Part model, mm, in its own coordinate system. Face numbers are marked on the shaded views. A direction names the side the tool comes from. Round coordinates to 2 decimals unless told otherwise and drop trailing zeros. Write each loop counter-clockwise with the first axis right and the second up, starting at its lowest first coordinate (ties: lowest second). Pieces come first, ordered by that corner, then holes. Notation, with made-up numbers: M -1,-37.5 L 55,-37.5 A17 cw 55,-27.5 Z; hole C -37,35 d5. An arc over 180 degrees is marked long. Answer as a JSON object with one key per item and string values. Group by question number.
1. Band-saw the part on D-D, the plane z = 25.5. Write the cut outline in (x, y).
2. Drop flat-ended pins along their axis: pin 1 (2 mm diameter, centred on x = -17.5, y = -7, fed in from +Z); pin 2 (1.5 mm diameter, centred on x = -1, z = 5.5, fed in from +Y); pin 3 (1.4 mm diameter, centred on y = 6.5, z = 31, fed in from -X); pin 4 (2.5 mm diameter, centred on x = -9.525, z = 15, fed in from -Y). Give the stop position or say it passes through.
3. Drill centre lines: line 1 (X direction, y = -4, z = 15) (3 decimals); line 2 (X direction, y = -14.25, z = 5) (3 decimals); line 3 (Y direction, x = -15, z = 6.75). Where is each one in solid material? Low to high. Write a range as from..to.
4. Band-saw the part on B-B, the plane x = 5. Write the cut outline in (y, z).
5. Band-saw the part on C-C, the plane y = -7. Write the cut outline in (x, z) (3 decimals).
6. Which spindle directions (+Z, -Z, +X, -X, +Y, -Y) get a long thin tool onto all of the face, cutting with end or side? Do the marked faces 4, 5, 6, 7 and 8. Say none if no direction does.
7. Band-saw the part on A-A, the plane y = 6. Write the cut outline in (x, z).
8. Two-plate mould, pull along X, no slides. Class the marked faces 1, 2 and 3: +X half, -X half, draft (parallel to the pull), parting line (faces both ways), or undercut.
from build123d import *

# Parameters (mm, degrees)
SKETCH2_W                 = 45
SKETCH2_H                 = 20
BOSS_EXTRUDE1_DEPTH       = 33
M4X0_7_TAPPED_HOLE1_D     = 3.3
SKETCH3_R                 = 7.5
CUT_EXTRUDE1_DEPTH        = 45
SKETCH4_R                 = 4
CUT_EXTRUDE2_DEPTH        = 10
M3X0_5_TAPPED_HOLE1_D     = 2.5
M3X0_5_TAPPED_HOLE1_DEPTH = 8.5
M3X0_5_TAPPED_HOLE1_TIP   = 0.751075774
SKETCH5_W                 = 4
SKETCH5_H                 = 1.5
CUT_EXTRUDE3_DEPTH        = 39
FILLET1_R                 = 9
SKETCH8_W                 = 15
SKETCH8_H                 = 4.75
BOSS_EXTRUDE2_DEPTH       = 7
M4X0_7_TAPPED_HOLE3_D     = 3.3
BODY_MOVE_COPY1_ANGLE     = 180


with BuildPart() as part:
    # Sketch2 → Boss-Extrude1 (new body)
    with BuildSketch(Plane.XY):
        Rectangle(SKETCH2_W, SKETCH2_H)
    extrude(amount=BOSS_EXTRUDE1_DEPTH)

    # M4x0.7 Tapped Hole1 (through all)
    with Locations(Plane(origin=(0, -10, 0), x_dir=(-1, 0, 0), z_dir=(0, -1, 0))):
        with Locations((-9.525, -15), (9.525, -15)):
            Hole(M4X0_7_TAPPED_HOLE1_D / 2)

    # Sketch3 → Cut-Extrude1 (cut)
    with BuildSketch(Plane(origin=(22.5, 0, 0), x_dir=(0, 0, -1), z_dir=(1, 0, 0))):
        with Locations((-30, 0)):
            Circle(SKETCH3_R)
    extrude(amount=-CUT_EXTRUDE1_DEPTH, mode=Mode.SUBTRACT)

    # Sketch4 → Cut-Extrude2 (cut)
    with BuildSketch(Plane(origin=(0, 0, 0), x_dir=(-1, 0, 0), z_dir=(0, 0, -1))):
        with Locations((-15, 0)):
            Circle(SKETCH4_R)
        with Locations((15, 0)):
            Circle(SKETCH4_R)
    extrude(amount=-CUT_EXTRUDE2_DEPTH, mode=Mode.SUBTRACT)

    # M3x0.5 Tapped Hole1
    with Locations(Plane(origin=(0, 10, 0), x_dir=(1, 0, 0), z_dir=(0, 1, 0))):
        with Locations((9.525, -5), (-9.525, -5)):
            Hole(M3X0_5_TAPPED_HOLE1_D / 2, depth=M3X0_5_TAPPED_HOLE1_DEPTH)
            with Locations((0, 0, -(M3X0_5_TAPPED_HOLE1_DEPTH + M3X0_5_TAPPED_HOLE1_TIP / 2))):  # 118° drill point
                Cone(0, M3X0_5_TAPPED_HOLE1_D / 2, M3X0_5_TAPPED_HOLE1_TIP, mode=Mode.SUBTRACT)

    # Sketch5 → Cut-Extrude3 (cut)
    with BuildSketch(Plane.XZ.offset(10)):
        with Locations((-17, 20.25)):
            Rectangle(SKETCH5_W, SKETCH5_H)
        with Locations((17, 20.25)):
            Rectangle(SKETCH5_W, SKETCH5_H)
    extrude(amount=-CUT_EXTRUDE3_DEPTH, mode=Mode.SUBTRACT)

    # Fillet1
    fillet1_edges = [part.edges().sort_by_distance(p)[0] for p in [
        (-17, -10, 21),
        (17, -10, 21),
    ]]
    fillet(fillet1_edges, radius=FILLET1_R)

    # Sketch8 → Boss-Extrude2 (add)
    with BuildSketch(Plane.XZ.offset(10)):
        with Locations((0, 30.625)):
            Rectangle(SKETCH8_W, SKETCH8_H)
    extrude(amount=BOSS_EXTRUDE2_DEPTH)

    # M4x0.7 Tapped Hole3 (through all)
    with Locations(Plane(origin=(0, 0, 28.25), x_dir=(-1, 0, 0), z_dir=(0, 0, -1))):
        with Locations((0, -13)):
            Hole(M4X0_7_TAPPED_HOLE3_D / 2)


with BuildPart() as part_1:
    # Body-Move/Copy1: moved
    add(part.part.rotate(Axis((0, -3.5, 0), (0, 0, 1)), BODY_MOVE_COPY1_ANGLE))


solid = part_1.part
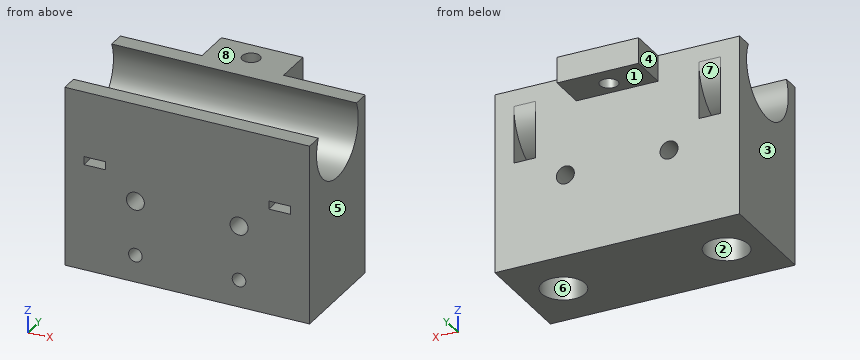
Worked answers:
{
 "1": {"outline": "M -22.5,-17 L 22.5,-17 L 22.5,-13 L -22.5,-13 Z; M -22.5,-1 L 22.5,-1 L 22.5,3 L 19,3 L 19,1.79 L 15,1.79 L 15,3 L -15,3 L -15,1.79 L -19,1.79 L -19,3 L -22.5,3 Z"},
 "2": {"pin 1": "stops at z = 22.57", "pin 2": "stops at y = 3", "pin 3": "stops at x = -7.5", "pin 4": "passes through"},
 "3": {"line 1": "x = -22.5..-11.175, -7.875..7.875, 11.175..22.5", "line 2": "x = -22.5..-10.775, -8.275..8.275, 10.775..22.5", "line 3": "y = -17..-11, -3..3"},
 "4": {"outline": "M -17,0 L 3,0 L 3,28.25 L 10,28.25 L 10,33 L -0.13,33 A7.5 cw long -13.87,33 L -17,33 Z"},
 "5": {"outline": "M -22.5,0 L -19,0 L -19,10 L -11,10 L -11,0 L 11,0 L 11,10 L 19,10 L 19,0 L 22.5,0 L 22.5,22.5 L -22.5,22.5 Z; hole M -19,19.5 L -15,19.5 L -15,21 L -19,21 Z; hole C -9.525,15 d3.3; hole C 9.525,15 d3.3; hole M 15,19.5 L 19,19.5 L 19,21 L 15,21 Z"},
 "6": {"face 4": "+Z, -Z, -X, +Y", "face 5": "+Z, -Z, +X, +Y, -Y", "face 6": "-Z", "face 7": "+Y", "face 8": "+Z, +X, -X, +Y, -Y"},
 "7": {"outline": "M -7.5,28.25 L -1.65,28.25 L -1.65,33 L -7.5,33 Z; M 1.65,28.25 L 7.5,28.25 L 7.5,33 L 1.65,33 Z"},
 "8": {"face 1": "draft", "face 2": "undercut", "face 3": "-X half"}
}
